```python
from build123d import *

# Parameters (mm, degrees)
SKETCH1_R             = 12.5
BOSS_EXTRUDE1_DEPTH   = 23
SKETCH2_R             = 3.5
BOSS_EXTRUDE2_DEPTH   = 2.5
SKETCH3_R             = 2
BOSS_EXTRUDE4_DEPTH   = 9.5
SKETCH4_W             = 2.645751312
SKETCH4_H             = 0.5
CUT_EXTRUDE1_DEPTH    = 8
SKETCH5_R             = 12.2
BOSS_EXTRUDE5_DEPTH   = 31
SKETCH6_R             = 3.2
BOSS_EXTRUDE6_DEPTH   = 1.4
SKETCH7_W             = 0.5
SKETCH7_H             = 2
BOSS_EXTRUDE7_DEPTH   = 3.1
M3_TAPPED_HOLE1_D     = 2.5
M3_TAPPED_HOLE1_DEPTH = 8.5
M3_TAPPED_HOLE1_TIP   = 0.751075774


with BuildPart() as part:
    # Sketch1 → Boss-Extrude1 (new body)
    with BuildSketch(Plane.XY):
        Circle(SKETCH1_R)
    extrude(amount=-BOSS_EXTRUDE1_DEPTH)

    # Sketch2 → Boss-Extrude2 (add)
    with BuildSketch(Plane.XY):
        Circle(SKETCH2_R)
    extrude(amount=BOSS_EXTRUDE2_DEPTH)

    # Sketch3 → Boss-Extrude4 (add)
    with BuildSketch(Plane.XY.offset(2.5)):
        Circle(SKETCH3_R)
    extrude(amount=BOSS_EXTRUDE4_DEPTH)

    # Sketch4 → Cut-Extrude1 (cut)
    with BuildSketch(Plane.XY.offset(12)):
        with Locations((0, 1.75)):
            Rectangle(SKETCH4_W, SKETCH4_H)
    extrude(amount=-CUT_EXTRUDE1_DEPTH, mode=Mode.SUBTRACT)

    # Sketch5 → Boss-Extrude5 (add)
    with BuildSketch(Plane(origin=(0, 0, -23), x_dir=(-1, 0, 0), z_dir=(0, 0, -1))):
        with Locations(Location((0, 0, 0), (0, 0, 180))):
            Circle(SKETCH5_R)
    extrude(amount=BOSS_EXTRUDE5_DEPTH)

    # Sketch6 → Boss-Extrude6 (add)
    with BuildSketch(Plane(origin=(0, 0, -54), x_dir=(-1, 0, 0), z_dir=(0, 0, -1))):
        Circle(SKETCH6_R)
    extrude(amount=BOSS_EXTRUDE6_DEPTH)

    # Sketch7 → Boss-Extrude7 (add)
    with BuildSketch(Plane(origin=(0, 0, -54), x_dir=(-1, 0, 0), z_dir=(0, 0, -1))):
        with Locations((0, 8.5)):
            Rectangle(SKETCH7_W, SKETCH7_H)
        with Locations((0, -8.5)):
            Rectangle(SKETCH7_W, SKETCH7_H)
    extrude(amount=BOSS_EXTRUDE7_DEPTH)

    # M3 Tapped Hole1
    with Locations(Plane.XY):
        with Locations((0, 8.5), (0, -8.5)):
            Hole(M3_TAPPED_HOLE1_D / 2, depth=M3_TAPPED_HOLE1_DEPTH)
            with Locations((0, 0, -(M3_TAPPED_HOLE1_DEPTH + M3_TAPPED_HOLE1_TIP / 2))):  # 118° drill point
                Cone(0, M3_TAPPED_HOLE1_D / 2, M3_TAPPED_HOLE1_TIP, mode=Mode.SUBTRACT)


solid = part.part
```
Verification items for the finished model (mm, model axes). A direction names the side the tool comes from. Give positions to 0.01 mm unless a question says otherwise; leave off trailing zeros. Order: outer loops, then holes, each group sorted by start corner. A loop starts at its lowest first (then second) coordinate and runs counter-clockwise, first axis right, second up. Notation, with made-up numbers: M 20.5,51 L 28.5,51 A13 cw 28.5,61 Z; hole C -29,24 d9. An arc over 180 degrees is marked long. Return JSON: item names as keys, results as strings. Group by question number.
1) Access from +Z, -Z, +X, -X, +Y, -Y to the whole of each face (thin tool, end or side, straight path). Record for faces 4 (the face through (0, 0, -55.4)), 5 (the face through (2.539, -1.947, -54.69)), 6 (the face through (3, -3, 0)).
2) Section check B-B on x = -4.25. Record the cut outline in (y, z).
3) Go/stop test with flat-tipped pins: pin 1 Ø12.5 at (x, y) = (0, 1) entering from -Z; pin 2 Ø8 at (y, z) = (-4.5, -16) entering from -X; pin 3 Ø6 at (x, z) = (-8.5, -46.5) entering from +Y. Record where each tip stops, or that it passes through.
4) Scan lines: line 1 (Y direction, x = 0, z = -5.75); line 2 (Z direction, x = 7.25, y = -4.25); line 3 (X direction, y = 8.5, z = -5.5). Record each from-to range of solid material in increasing order.
5) Section check A-A on y = 0. Record the cut outline in (x, z), and give its area (3 significant figures).
6) Mould release check, pull along Y, two halves, no side actions. Record for faces 1 (the face through (3.233, -1.341, 1.232)), 2 (the face through (0.2, -8.58, -9.12)), 3 (the face through (-0.25, -9, -56)): pulls with the +Y half, pulls with the -Y half, needs draft (parallel to the pull), parting line crosses it, or undercut.
7) Section check D-D on z = -42. Record the cut outline in (x, y).
8) Section check C-C on z = 7.5. Record the cut outline in (x, y), and give its area (3 significant figures).
Answer block:
{
 "1": {"face 4": "-Z, +X, -X", "face 5": "-Z", "face 6": "+Z"},
 "2": {"outline": "M -11.76,-23 L -11.44,-23 L -11.44,-54 L 11.44,-54 L 11.44,-23 L 11.76,-23 L 11.76,0 L -11.76,0 Z"},
 "3": {"pin 1": "stops at z = -55.4", "pin 2": "stops at x = -12.49", "pin 3": "stops at y = 10.89"},
 "4": {"line 1": "y = -12.5 to -9.75, -7.25 to 7.25, 9.75 to 12.5", "line 2": "z = -54 to 0", "line 3": "x = -9.17 to -1.25, 1.25 to 9.17"},
 "5": {"outline": "M -12.5,-23 L -12.2,-23 L -12.2,-54 L -3.2,-54 L -3.2,-55.4 L 3.2,-55.4 L 3.2,-54 L 12.2,-54 L 12.2,-23 L 12.5,-23 L 12.5,0 L 3.5,0 L 3.5,2.5 L 2,2.5 L 2,12 L -2,12 L -2,2.5 L -3.5,2.5 L -3.5,0 L -12.5,0 Z", "area": "1,400 mm^2"},
 "6": {"face 1": "parting line crosses it", "face 2": "undercut", "face 3": "needs draft"},
 "7": {"outline": "C 0,0 d24.4"},
 "8": {"outline": "M -1.32,1.5 A2 ccw long 1.32,1.5 Z", "area": "11.7 mm^2"}
}
